Design review of the part built by this model. Coordinates are the model's own, in mm. Face numbers are marked on the shaded views. A direction names the side the tool comes from. Give positions to 0.01 mm unless a question says otherwise; leave off trailing zeros. Order: outer loops, then holes, each group sorted by start corner. A loop starts at its lowest first (then second) coordinate and runs counter-clockwise, first axis right, second up. Notation, with made-up numbers: (8.5, 4.5) -> (31.5, 4.5) arc R19 ccw to (31.5, 36.5) -> close; hole circle Ø9 at (11, 19). An arc over 180 degrees is marked (long way). Return JSON: item names as keys, results as strings.
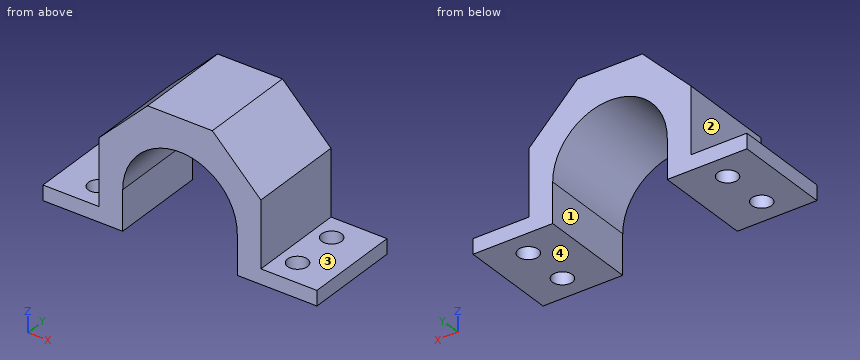
```python
from build123d import *

# Parameters (mm, degrees)
BOSS_EXTRUDE1_DEPTH = 39
SKETCH2_R           = 4
CUT_EXTRUDE1_DEPTH  = 53


with BuildPart() as part:
    # Sketch1 → Boss-Extrude1 (new body)
    with BuildSketch(Plane(origin=(0, 0, 0), x_dir=(1, 0, 0), z_dir=(0, 1, 0))):
        with BuildLine():
            Line((-23, 0), (-23, 10))
            Line((-23, 10), (-23, 16))
            Line((-23, 16), (-55, 16))
            Line((-55, 16), (-55, 10))
            Line((-55, 10), (-32.5, 10))
            Line((-32.5, 10), (-32.5, -16.5))
            Line((-32.5, -16.5), (-13, -36))
            Line((-13, -36), (13, -36))
            Line((13, -36), (32.5, -16.5))
            Line((32.5, -16.5), (32.5, 10))
            Line((32.5, 10), (55, 10))
            Line((55, 10), (55, 16))
            Line((55, 16), (23, 16))
            Line((23, 16), (23, 10))
            Line((23, 10), (23, 0))
            ThreePointArc((23, 0), (0, -23), (-23, 0))
        make_face()
    extrude(amount=BOSS_EXTRUDE1_DEPTH)

    # Sketch2 → Cut-Extrude1 (cut, through all)
    with BuildSketch(Plane(origin=(0, 0, -16), x_dir=(-1, 0, 0), z_dir=(0, 0, -1))):
        with Locations((-40, 29)):
            Circle(SKETCH2_R)
        with Locations((-40, 10)):
            Circle(SKETCH2_R)
        with Locations((40, 29)):
            Circle(SKETCH2_R)
        with Locations((40, 10)):
            Circle(SKETCH2_R)
    extrude(amount=-CUT_EXTRUDE1_DEPTH, mode=Mode.SUBTRACT)


solid = part.part
```
Item 1: For pin 1 (21 mm diameter, centred on y = 19, z = 3.5, fed in from -X); pin 2 (7 mm diameter, centred on x = 47, y = 18.5, fed in from +Z); pin 3 (8 mm diameter, centred on y = 25, z = 8.5, fed in from +X); pin 4 (12 mm diameter, centred on y = 30.5, z = -7.5, fed in from -X), all flat-tipped, find the tip position at first contact; note any pin that passes through.
Result set:
{"pin 1": "stops at x = -32.5", "pin 2": "stops at z = -10", "pin 3": "stops at x = 32.5", "pin 4": "stops at x = -55"}
Item 2: Add section A-A (y = 29). Give the boundary of the cut face in (x, z).
Result set:
{"outline": "(-55, -16) -> (-44, -16) -> (-44, -10) -> (-55, -10) -> close; (-36, -16) -> (-23, -16) -> (-23, 0) arc R23 cw to (23, 0) -> (23, -16) -> (36, -16) -> (36, -10) -> (32.5, -10) -> (32.5, 16.5) -> (13, 36) -> (-13, 36) -> (-32.5, 16.5) -> (-32.5, -10) -> (-36, -10) -> close; (44, -16) -> (55, -16) -> (55, -10) -> (44, -10) -> close"}
Item 3: Add section D-D (y = 20). Give the boundary of the cut face in (x, z).
Result set:
{"outline": "(-55, -16) -> (-23, -16) -> (-23, 0) arc R23 cw to (23, 0) -> (23, -16) -> (55, -16) -> (55, -10) -> (32.5, -10) -> (32.5, 16.5) -> (13, 36) -> (-13, 36) -> (-32.5, 16.5) -> (-32.5, -10) -> (-55, -10) -> close"}
Item 4: Wall thickness on L1, parallel to Y at x = -40, z = -12; L2, parallel to X at y = 22, z = -7; L3, parallel to Z at x = -0.5, y = 18.5: over which ranges is each line inside the solid? List them lowest first. Write a range as [from, to].
Result set:
{"L1": "y = [0, 6], [14, 25], [33, 39]", "L2": "x = [-32.5, -23], [23, 32.5]", "L3": "z = [22.99, 36]"}
Item 5: Add section B-B (x = 40). Give the boundary of the cut face in (y, z), plus the area to 3 significant figures.
Result set:
{"outline": "(0, -16) -> (6, -16) -> (6, -10) -> (0, -10) -> close; (14, -16) -> (25, -16) -> (25, -10) -> (14, -10) -> close; (33, -16) -> (39, -16) -> (39, -10) -> (33, -10) -> close", "area": "138 mm^2"}
Item 6: Add section C-C (z = 11). Give the boundary of the cut face in (x, y), plus the area to 3 significant figures.
Result set:
{"outline": "(-32.5, 0) -> (-20.2, 0) -> (-20.2, 39) -> (-32.5, 39) -> close; (20.2, 0) -> (32.5, 0) -> (32.5, 39) -> (20.2, 39) -> close", "area": "959 mm^2"}
Item 7: Machinability: for the marked faces 1, 2, 3 and 4, which of the approach directions +Z, -Z, +X, -X, +Y, -Y give a long, thin tool a straight path to every point of the face, cutting with its end or side? Answer none if there is none.
Result set:
{"face 1": "-Z, +Y, -Y", "face 2": "+Z, -X, +Y, -Y", "face 3": "+Z, +X, +Y, -Y", "face 4": "-Z, +X, -X, +Y, -Y"}
